from build123d import *

# Parameters (mm, degrees)
SKETCH1_W           = 100
SKETCH1_H           = 63.5
BOSS_EXTRUDE1_DEPTH = 3
SKETCH2_W           = 12.5
SKETCH2_H           = 3
SKETCH2_W_2         = 15
CUT_EXTRUDE1_DEPTH  = 4


with BuildPart() as part:
    # Sketch1 → Boss-Extrude1 (new body)
    with BuildSketch(Plane.XY):
        Rectangle(SKETCH1_W, SKETCH1_H)
    extrude(amount=BOSS_EXTRUDE1_DEPTH)

    # Sketch2 → Cut-Extrude1 (cut, through all)
    with BuildSketch(Plane.XY.offset(3)):
        with Locations((-43.75, 30.25)):
            Rectangle(SKETCH2_W, SKETCH2_H)
        with Locations((-15, 30.25)):
            Rectangle(SKETCH2_W_2, SKETCH2_H)
        with Locations((15, 30.25)):
            Rectangle(SKETCH2_W_2, SKETCH2_H)
        with Locations((43.75, 30.25)):
            Rectangle(SKETCH2_W, SKETCH2_H)
    cut_extrude1 = extrude(amount=-CUT_EXTRUDE1_DEPTH, mode=Mode.SUBTRACT)

    # Mirror2: Cut-Extrude1 across plane
    add(cut_extrude1.mirror(Plane.ZX), mode=Mode.SUBTRACT)


solid = part.part
The model under review builds one solid part; all positions refer to its coordinate system, in mm. A direction names the side the tool comes from. Round coordinates to 2 decimals unless told otherwise and drop trailing zeros. Loops run counter-clockwise (first coordinate to the right, second up) from the corner with the lowest first, then second, coordinate; pieces in that order, holes last. Notation, with made-up numbers: M 59.5,68.25 L 79.5,68.25 A9 cw 79.5,78.25 Z; hole C 70,20.25 d11. An arc over 180 degrees is marked long. Answer as a JSON object with one key per item and string values.
Item 1: Tool access review of faces 1 (the face through (-37.5, -30, 2)), 2 (the face through (22.5, 30, 2)), 3 (the face through (44, -28.75, 2)): name each direction out of +Z, -Z, +X, -X, +Y, -Y from which nothing blocks a thin tool from reaching the whole face with its end or side.
Check sheet entries:
{"face 1": "+Z, -Z, -X, -Y", "face 2": "+Z, -Z, +Y", "face 3": "+Z, -Z, +X, -Y"}
Item 2: The part is to be moulded in two halves that separate along X. For faces 4 (the face through (50, 0, 1)), 5 (the face through (-30, -31.75, 1)), 6 (the face through (22.5, -30, 2)), say which applies: +X half, -X half, draft (parallel to the pull), parting line (faces both ways), or undercut.
Check sheet entries:
{"face 4": "+X half", "face 5": "draft", "face 6": "undercut"}
Item 3: We need section B-B, the plane x = -19. State the section outline as (y, z) points.
Check sheet entries:
{"outline": "M -28.75,0 L 28.75,0 L 28.75,3 L -28.75,3 Z"}
Item 4: For line 1 along Y through (x, z) = (19, 0.95), list the stretches that pass through material, from the lowest coordinate up.
Check sheet entries:
{"line 1": "-28.75 to 28.75"}
Item 5: Clearance check with flat-ended pins moving along their axes: P1, Ø1.5, axis at x = 38.5, z = 2.5, coming from the +Y side; P2, Ø3, axis at x = 37.5, y = 12.5, coming from the -Z side; P3, Ø0.9, axis at y = 31, z = 2, coming from the +X side; P4, Ø1.5, axis at x = 13, z = 1, coming from the -Y side. State where each tip first meets the part, or that it passes through.
Check sheet entries:
{"P1": "y = 28.75", "P2": "z = 0", "P3": "x = 37.5", "P4": "y = -28.75"}
Item 6: We need section A-A, the plane z = 2.05. State the section outline as (x, y) points.
Check sheet entries:
{"outline": "M -50,-28.75 L -37.5,-28.75 L -37.5,-31.75 L -22.5,-31.75 L -22.5,-28.75 L -7.5,-28.75 L -7.5,-31.75 L 7.5,-31.75 L 7.5,-28.75 L 22.5,-28.75 L 22.5,-31.75 L 37.5,-31.75 L 37.5,-28.75 L 50,-28.75 L 50,28.75 L 37.5,28.75 L 37.5,31.75 L 22.5,31.75 L 22.5,28.75 L 7.5,28.75 L 7.5,31.75 L -7.5,31.75 L -7.5,28.75 L -22.5,28.75 L -22.5,31.75 L -37.5,31.75 L -37.5,28.75 L -50,28.75 Z"}
